CAD build for the part. Positions are in the model's coordinates, mm. A direction names the side the tool comes from. Give positions to 0.01 mm unless a question says otherwise; leave off trailing zeros. Loops run counter-clockwise (first coordinate to the right, second up) from the corner with the lowest first, then second, coordinate; pieces in that order, holes last. Notation, with made-up numbers: (86, 12.25) - (136, 12.25) arc R29 ccw to (136, 44.25) - close; hole circle Ø9 at (26, 39.25). An arc over 180 degrees is marked (long way). Return JSON: item names as keys, results as strings.
from build123d import *

# Parameters (mm, degrees)
EXTRUDE_1_DEPTH     = 20
SKETCH_4_W          = 34
SKETCH_4_H          = 20
EXTRUDE_2_DEPTH     = 2
SKETCH_5_R          = 6.5
EXTRUDE_3_DEPTH     = 1.5
SKETCH_6_R          = 2.75
EXTRUDE_4_DEPTH     = 4
SKETCH_7_R          = 2
CUT_EXTRUDE_1_DEPTH = 44.324617713


with BuildPart() as part:
    # 草图3 → 凸台-拉伸1 (new body)
    with BuildSketch(Plane.XY):
        Polygon((-20.35, 16.655405405), (20.35, 16.655405405), (20.35, -10.344594595), (27.35, -10.344594595), (27.35, -12.844594595), (20.35, -12.844594595), (20.35, -18.844594595), (-20.35, -18.844594595), (-20.35, -12.844594595), (-27.35, -12.844594595), (-27.35, -10.344594595), (-20.35, -10.344594595), align=None)
    extrude(amount=EXTRUDE_1_DEPTH)

    # 草图4 → 凸台-拉伸2 (add)
    with BuildSketch(Plane.XZ.offset(18.844594595)):
        with Locations((-3.35, 10)):
            Rectangle(SKETCH_4_W, SKETCH_4_H)
    extrude(amount=EXTRUDE_2_DEPTH)

    # 草图5 → 凸台-拉伸3 (add)
    with BuildSketch(Plane.XZ.offset(20.844594595)):
        with Locations(Location((-10.364971528, 10, 0), (0, 0, 270))):
            Circle(SKETCH_5_R)
    extrude(amount=EXTRUDE_3_DEPTH)

    # 草图6 → 凸台-拉伸4 (add)
    with BuildSketch(Plane.XZ.offset(22.344594595)):
        with Locations(Location((-10.364971528, 10, 0), (0, 0, 270))):
            Circle(SKETCH_6_R)
    extrude(amount=EXTRUDE_4_DEPTH)

    # 草图7 → 切除-拉伸1 (cut, through all)
    with BuildSketch(Plane(origin=(0, -10.344594595, 0), x_dir=(1, 0, 0), z_dir=(0, 1, 0))):
        with Locations(Location((-24.315, -4.993540971, 0), (0, 0, 270))):
            Circle(SKETCH_7_R)
        with Locations(Location((24.315, -4.993540971, 0), (0, 0, 270))):
            Circle(SKETCH_7_R)
        with Locations(Location((24.315, -14.993540971, 0), (0, 0, 270))):
            Circle(SKETCH_7_R)
        with Locations(Location((-24.315, -14.993540971, 0), (0, 0, 180))):
            Circle(SKETCH_7_R)
    extrude(amount=-CUT_EXTRUDE_1_DEPTH, mode=Mode.SUBTRACT)


solid = part.part
1. Cut at D-D, the plane z = 10. Write the cut outline in (x, y), plus the area to 3 significant figures.
Values follow:
{"outline": "(-27.35, -12.84) - (-20.35, -12.84) - (-20.35, -20.84) - (-16.86, -20.84) - (-16.86, -22.34) - (-13.11, -22.34) - (-13.11, -26.34) - (-7.61, -26.34) - (-7.61, -22.34) - (-3.86, -22.34) - (-3.86, -20.84) - (13.65, -20.84) - (13.65, -18.84) - (20.35, -18.84) - (20.35, -12.84) - (27.35, -12.84) - (27.35, -10.34) - (20.35, -10.34) - (20.35, 16.66) - (-20.35, 16.66) - (-20.35, -10.34) - (-27.35, -10.34) - close", "area": "1,590 mm²"}
2. Which spindle directions (+Z, -Z, +X, -X, +Y, -Y) get a long thin tool onto all of the face, cutting with end or side? Do faces 1 (the face through (13.65, -20, 10)), 2 (the face through (-20.35, 3, 10)), 3 (the face through (-10, -22.345, 7)). Say none if no direction does.
Values follow:
{"face 1": "+Z, -Z, +X, -Y", "face 2": "+Z, -Z, -X, +Y", "face 3": "-Y"}
3. Cut at C-C, the plane y = 0. Write the cut outline in (x, z), plus the area to 3 significant figures.
Values follow:
{"outline": "(-20.35, 0) - (20.35, 0) - (20.35, 20) - (-20.35, 20) - close", "area": "814 mm²"}
4. Drop flat-ended pins along their axis: P1, Ø10, axis at y = 5.5, z = 8.5, coming from the +X side; P2, Ø1, axis at y = 4, z = 5.5, coming from the -X side; P3, Ø4.5, axis at x = -24.32, z = 14.99, coming from the +Y side. Give the stop position or say it passes through.
Values follow:
{"P1": "stops at x = 20.35", "P2": "stops at x = -20.35", "P3": "stops at y = -10.34"}
5. Drill centre lines: probe 1 along X at (y, z) = (7.5, 3.75); probe 2 along Y at (x, z) = (-4.5, 10.25); probe 3 along Y at (x, z) = (6.5, 11). Where is each one in solid material? Low to high.
Values follow:
{"probe 1": "x = -20.35 to 20.35", "probe 2": "y = -22.34 to 16.66", "probe 3": "y = -20.84 to 16.66"}
6. Cut at A-A, the plane z = 18. Write the cut outline in (x, y).
Values follow:
{"outline": "(-27.35, -12.84) - (-20.35, -12.84) - (-20.35, -20.84) - (13.65, -20.84) - (13.65, -18.84) - (20.35, -18.84) - (20.35, -12.84) - (27.35, -12.84) - (27.35, -10.34) - (20.35, -10.34) - (20.35, 16.66) - (-20.35, 16.66) - (-20.35, -10.34) - (-27.35, -10.34) - close"}
7. Cut at B-B, the plane x = -6.5. Write the cut outline in (y, z), plus the area to 3 significant figures.
Values follow:
{"outline": "(-22.34, 4.77) - (-20.84, 4.77) - (-20.84, 0) - (16.66, 0) - (16.66, 20) - (-20.84, 20) - (-20.84, 15.23) - (-22.34, 15.23) - close", "area": "766 mm²"}
8. Pull direction Z, two halves, no side cores. Call faces 4 (the face through (-8.046, -24.317, 8.522)), 5 (the face through (24.92, -11.58, 6.9)), 6 (the face through (-26.162, -11.577, 14.228)), 7 (the face through (0, -2, 0)): +Z half, -Z half, draft (parallel to the pull), parting line (faces both ways), or undercut.
Values follow:
{"face 4": "parting line", "face 5": "undercut", "face 6": "undercut", "face 7": "-Z half"}
